Verification items for the finished model (mm, model axes). A direction names the side the tool comes from. Round coordinates to 2 decimals unless told otherwise and drop trailing zeros. Order: outer loops, then holes, each group sorted by start corner. A loop starts at its lowest first (then second) coordinate and runs counter-clockwise, first axis right, second up. Notation, with made-up numbers: (3.25, -28) -> (55.25, -28) arc R20 ccw to (55.25, -11) -> close; hole circle Ø5 at (39, -10.75). An arc over 180 degrees is marked (long way). Return JSON: item names as keys, results as strings. Group by question number.
1) Depth check by flat-ended pin: pin 1 (5 mm diameter, centred on x = 8, z = 8, fed in from +Y); pin 2 (8 mm diameter, centred on x = -5, z = 7.5, fed in from +Y); pin 3 (2 mm diameter, centred on x = 4.5, z = 19, fed in from +Y). Enter the tip coordinate at first touch or a pass-through.
2) Section check A-A on y = 4. Enter the section's corners in (x, z), plus the area to 3 significant figures.
3) Draft check along X on faces 5 (the flat face through (16.54, 6.66, 19.72)), 6 (the flat face through (-16.46, 6.84, 19.72)), 7 (the flat face through (7.5, 0, 20)). Enter one of: pulls with the +X half, pulls with the -X half, needs draft (parallel to the pull), parting line crosses it, or undercut.
4) Tool access check on faces 1 (the flat face through (4.98, -10.54, 32.4)), 2 (the flat face through (-6.656, 15.528, 19.72)), 3 (the flat face through (3.5, -10, 12)), 4 (the flat face through (-5, -7.5, 15)). Record the directions out of +Z, -Z, +X, -X, +Y, -Y that give a thin tool (end or side, any length) a straight path to the whole face; none if there is none.
5) Scan lines: L1, parallel to X at y = 2, z = 24; L2, parallel to X at y = -4, z = 13; L3, parallel to Y at x = 6.5, z = 11.5. Record each from-to range of solid material in increasing order.
6) Section check D-D on x = -14.5. Enter the section's corners in (y, z), plus the area to 3 significant figures.
7) Section check C-C on y = -6. Enter the section's corners in (x, z), plus the area to 3 significant figures.
8) Section check B-B on z = 29. Enter the section's corners in (x, y).
```python
from build123d import *

# Parameters (mm, degrees)
F1_DEPTH = 40
F3_DEPTH = 6


with BuildPart() as f1:
    # F0 (on Top) → F1 (new body)
    with BuildSketch(Plane.XY):
        Polygon((-7.5, -7.5), (-7.5, 7.5), (7.5, 7.5), (7.5, -7.5), (3.5, -7.5), (3.5, -13.5), (13.5, -13.5), (19.5, 0), (13.5, 13.5), (0, 17.5), (-13.5, 13.5), (-19.5, 0), (-13.5, -13.5), (-3.5, -13.5), (-3.5, -7.5), align=None)
    extrude(amount=F1_DEPTH)

    # F2 (on face) → F3 (cut)
    with BuildSketch(Plane.XZ.offset(13.5)):
        Polygon((-3.5, 25), (-3.5, 40), (-6.5, 40), align=None)
        Polygon((3.5, 25), (6.5, 40), (3.5, 40), align=None)
    extrude(amount=-F3_DEPTH, mode=Mode.SUBTRACT)


solid = f1.part
```
Check result:
{
 "1": {"pin 1": "y = 15.87", "pin 2": "y = 17.2", "pin 3": "y = 16.46"},
 "2": {"outline": "(-17.72, 0) -> (-7.5, 0) -> (-7.5, 40) -> (-17.72, 40) -> close; (7.5, 0) -> (17.72, 0) -> (17.72, 40) -> (7.5, 40) -> close", "area": "818 mm^2"},
 "3": {"face 5": "pulls with the +X half", "face 6": "pulls with the -X half", "face 7": "undercut"},
 "4": {"face 1": "+Z, -Y", "face 2": "+Z, -Z, -X, +Y", "face 3": "+Z, -Z, -Y", "face 4": "+Z, -Z"},
 "5": {"L1": "-18.61 to -7.5, 7.5 to 18.61", "L2": "-17.72 to -7.5, 7.5 to 17.72", "L3": "-13.5 to -7.5, 7.5 to 15.57"},
 "6": {"outline": "(-11.25, 0) -> (11.25, 0) -> (11.25, 40) -> (-11.25, 40) -> close", "area": "900 mm^2"},
 "7": {"outline": "(-16.83, 0) -> (-7.5, 0) -> (-7.5, 40) -> (-16.83, 40) -> close; (7.5, 0) -> (16.83, 0) -> (16.83, 40) -> (7.5, 40) -> close", "area": "747 mm^2"},
 "8": {"outline": "(-19.5, 0) -> (-13.5, -13.5) -> (-4.3, -13.5) -> (-4.3, -7.5) -> (-7.5, -7.5) -> (-7.5, 7.5) -> (7.5, 7.5) -> (7.5, -7.5) -> (4.3, -7.5) -> (4.3, -13.5) -> (13.5, -13.5) -> (19.5, 0) -> (13.5, 13.5) -> (0, 17.5) -> (-13.5, 13.5) -> close"}
}
